Part print with two shaded views. Sizes in mm from the minimum x, y, z corner. A direction names the side the tool comes from. Coordinates: 2 decimals unless noted, no trailing zeros. Loops run counter-clockwise (first coordinate to the right, second up) from the corner with the lowest first, then second, coordinate; pieces in that order, holes last.
(1) Tool access for the marked faces 5, 6 and 7: list every direction of +Z, -Z, +X, -X, +Y, -Y with a clear straight run to the whole face (end or side of a thin tool).
(2) Slice it at A-A (z = 0.95). Give the cut face in (x, y) (3 decimals).
(3) Slice it at C-C (x = 4.5). Give the cut face in (y, z) (1 decimal), and give its area (3 significant figures).
(4) Flat gauge pins, fed straight in: P1, Ø0.6, axis at x = 3, y = 3.5, coming from the -Z side; P2, Ø2, axis at x = 8, y = 3.87, coming from the +Z side; P3, Ø1, axis at x = 4, y = 5, coming from the -Z side. Where does each tip first touch, or does it go through?
(5) Slice it at B-B (y = 2). Give the cut face in (x, z), and give its area (3 significant figures).
(6) Wall check: L1, parallel to X at y = 1, z = 0.4; L2, parallel to X at y = 3.5, z = 0.4; L3, parallel to X at y = 3.75, z = 2.6. Give the ranges that are in metal, low to high.
(7) Slice it at D-D (z = 4.7). Give the cut face in (x, y), and give its area (3 significant figures).
(8) Two-plate mould, pull along Y, no slides. Class the marked faces 1, 2, 3 and 4: pulls with the +Y half, pulls with the -Y half, needs draft (parallel to the pull), parting line crosses it, or undercut.
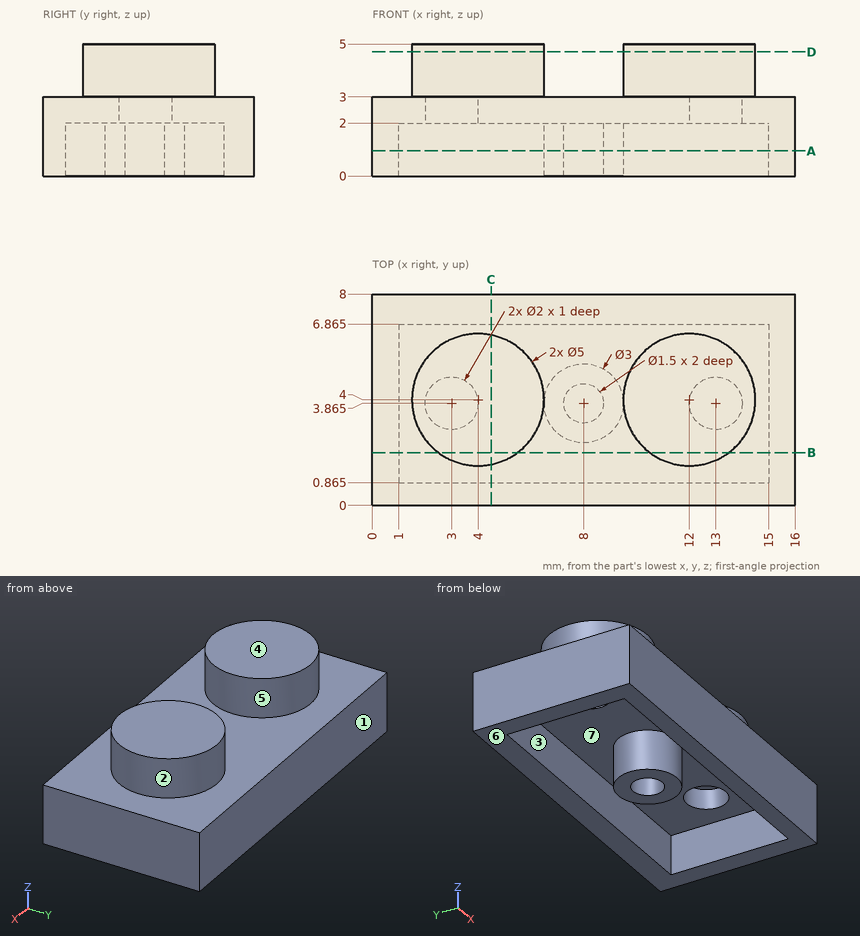
Response values:
1. face 5: +Z
1. face 6: -Z, +X, -X, +Y, -Y
1. face 7: -Z
2. outline: (0, 0) - (16, 0) - (16, 8) - (0, 8) - close; circle Ø3 at (8, 3.865); hole (1, 0.865) - (15, 0.865) - (15, 6.865) - (1, 6.865) - close; hole circle Ø1.5 at (8, 3.865)
3. outline: (0, 0) - (0.9, 0) - (0.9, 2) - (6.9, 2) - (6.9, 0) - (8, 0) - (8, 3) - (6.4, 3) - (6.4, 5) - (1.6, 5) - (1.6, 3) - (0, 3) - close
3. area: 21.8 mm2
4. P1: stops at z = 3
4. P2: stops at z = 3
4. P3: stops at z = 2
5. outline: (0, 0) - (1, 0) - (1, 2) - (15, 2) - (15, 0) - (16, 0) - (16, 3) - (13.5, 3) - (13.5, 5) - (10.5, 5) - (10.5, 3) - (5.5, 3) - (5.5, 5) - (2.5, 5) - (2.5, 3) - (0, 3) - close
5. area: 32.0 mm2
6. L1: x = 0 to 1, 15 to 16
6. L2: x = 0 to 1, 6.55 to 7.34, 8.66 to 9.45, 15 to 16
6. L3: x = 0 to 2.01, 3.99 to 12.01, 13.99 to 16
7. outline: circle Ø5 at (4, 4); circle Ø5 at (12, 4)
7. area: 39.3 mm2
8. face 1: pulls with the +Y half
8. face 2: parting line crosses it
8. face 3: undercut
8. face 4: needs draft
